Autodesk Inventor part; units mm, degrees
ref_plane "YZ Plane" through (0, 0, 0) normal (1, 0, 0) x (0, 1, 0)
ref_plane "XZ Plane" through (0, 0, 0) normal (0, 1, 0) x (-1, 0, 0)
ref_plane "XY Plane" through (0, 0, 0) normal (0, 0, 1) x (1, 0, 0)
sketch "スケッチ1" plane through (0, 0, 0) normal (0, 0, 1) x (1, 0, 0)
  circle A0 centre (0, 0) radius 6
  circle A1 centre (0, 0) radius 7
  dimension "d0" = 12
  dimension "d1" = 14
extrude "押し出し1" add sketch "スケッチ1" along normal blind 4
sketch "スケッチ2" plane through (0, 0, 0) normal (0, 0, -1) x (-1, 0, 0)
  circle A0 centre (0, 0) radius 7
  circle A1 centre (0, 0) radius 6
  circle A2 centre (0, 0) radius 10
  dimension "d4" = 20
extrude "押し出し2" add sketch "スケッチ2" along normal blind 1 contours A0 | A2
properties part number "オイレスフランジ付き12142004" material "アセタール樹脂、黒"
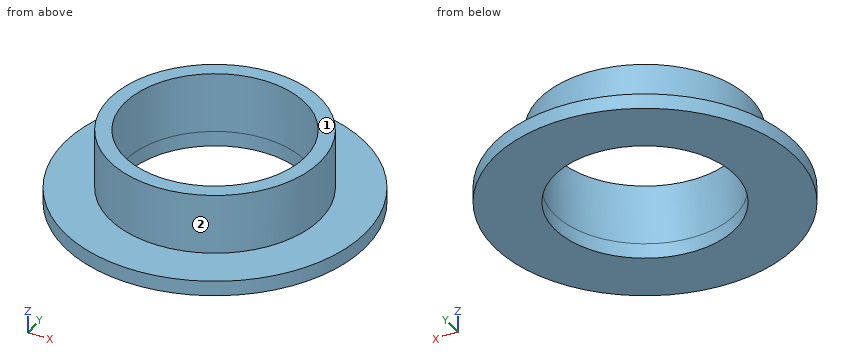
Verification items for the finished model (mm, model axes). Face numbers are marked on the shaded views. A direction names the side the tool comes from. Round coordinates to 2 decimals unless told otherwise and drop trailing zeros. Write each loop counter-clockwise with the first axis right and the second up, starting at its lowest first coordinate (ties: lowest second). Pieces come first, ordered by that corner, then holes. Notation, with made-up numbers: (-31.75, -27) - (19.25, -27) arc R24 cw to (19.25, 4) - close; hole circle Ø7 at (88.25, 71). An arc over 180 degrees is marked (long way). Answer as a JSON object with one key per item and string values. Group by question number.
Q1. Go/stop test with flat-tipped pins: pin 1 Ø2 at (x, z) = (1, 1.5) entering from -Y; pin 2 Ø6 at (x, y) = (2.5, -3.5) entering from +Z; pin 3 Ø7 at (x, y) = (0, 0) entering from +Z; pin 4 Ø1 at (x, z) = (5, 0) entering from +Y. Record where each tip stops, or that it passes through.
Q2. Thickness scan on line 1 (Y direction, x = 0.25, z = -0.1); line 2 (Y direction, x = 0, z = 2.1); line 3 (X direction, y = 1.5, z = 2.7). Record the ranges inside material, lowest first.
Q3. Section check A-A, the plane y = 0. Enter the section's corners in (x, z).
Q4. Section check D-D, the plane y = 6.5. Enter the section's corners in (x, z).
Q5. Section check C-C, the plane z = -0.5. Enter the section's corners in (x, y).
Q6. Tool access check on the marked faces 1 and 2. Record the directions out of +Z, -Z, +X, -X, +Y, -Y that give a thin tool (end or side, any length) a straight path to the whole face; none if there is none.
Found:
{
 "1": {"pin 1": "stops at y = -7", "pin 2": "stops at z = 4", "pin 3": "passes through", "pin 4": "stops at y = 8.93"},
 "2": {"line 1": "y = -10 to -5.99, 5.99 to 10", "line 2": "y = -7 to -6, 6 to 7", "line 3": "x = -6.84 to -5.81, 5.81 to 6.84"},
 "3": {"outline": "(-10, -1) - (-6, -1) - (-6, 4) - (-7, 4) - (-7, 0) - (-10, 0) - close; (6, -1) - (10, -1) - (10, 0) - (7, 0) - (7, 4) - (6, 4) - close"},
 "4": {"outline": "(-7.6, -1) - (7.6, -1) - (7.6, 0) - (2.6, 0) - (2.6, 4) - (-2.6, 4) - (-2.6, 0) - (-7.6, 0) - close"},
 "5": {"outline": "circle Ø20 at (0, 0); hole circle Ø12 at (0, 0)"},
 "6": {"face 1": "+Z, +X, -X, +Y, -Y", "face 2": "+Z"}
}
